Verification items for the finished model (mm, model axes). A direction names the side the tool comes from. Round coordinates to 2 decimals unless told otherwise and drop trailing zeros. Write each loop counter-clockwise with the first axis right and the second up, starting at its lowest first coordinate (ties: lowest second). Pieces come first, ordered by that corner, then holes. Notation, with made-up numbers: (63.25, 78) - (73.25, 78) arc R29 ccw to (73.25, 106) - close; hole circle Ø10 at (33, 79). An arc over 180 degrees is marked (long way). Answer as a JSON object with one key per item and string values. Group by question number.
1) Thickness scan on line 1 (Y direction, x = 34, z = 16.5); line 2 (X direction, y = -39, z = 21.5); line 3 (X direction, y = 39, z = 21.25). Record the ranges inside material, lowest first.
2) Go/stop test with flat-tipped pins: pin 1 Ø7 at (y, z) = (40, 12) entering from -X; pin 2 Ø1.9 at (y, z) = (-40.5, 14) entering from +X; pin 3 Ø12 at (x, y) = (20, -11) entering from +Z. Record where each tip stops, or that it passes through.
3) Set-up check for faces 1 (the flat face through (-1, 0, 15)), 2 (the flat face through (-40, 42, 15)), 3 (the flat face through (40, 42, 15)): record each of +Z, -Z, +X, -X, +Y, -Y from which the full face is reachable in a straight line by a thin tool's end or side.
4) Section check D-D (y = -14). Enter the section's corners in (x, z).
5) Mould release check, pull along Z, two halves, no side actions. Record for faces 4 (the cylindrical face through (59.47, -0.39, 7.4)), 5 (the cylindrical face through (29.514, -39.943, 20.304)), 6 (the flat face through (1, 1, 0)): +Z half, -Z half, draft (parallel to the pull), parting line (faces both ways), or undercut.
6) Section check C-C (x = 8). Enter the section's corners in (y, z).
7) Section check A-A (z = 18). Enter the section's corners in (x, y), then the cut area to 3 significant figures.
8) Section check B-B (x = -23). Enter the section's corners in (y, z).
```python
from build123d import *

# Parameters (mm, degrees)
SKETCH1_R               = 10.5
BOSS_EXTRUDE1_DEPTH     = 15
BOSS_EXTRUDE2_DEPTH     = 30
SKETCH2_R               = 2.25
CUT_EXTRUDE1_DEPTH      = 1
CUT_EXTRUDE1_DEPTH_BACK = 90.5


with BuildPart() as part:
    # Sketch1 → Boss-Extrude1 (new body)
    with BuildSketch(Plane.XY):
        with BuildLine():
            Line((-40.319533419, -35), (40.319533419, -35))
            ThreePointArc((40.319533419, -35), (42.786608734, -28.756118968), (47.370059804, -23.850562196))
            ThreePointArc((47.370059804, -23.850562196), (59.471288553, 0.00030559), (47.370059804, 23.851173376))
            ThreePointArc((47.370059804, 23.851173376), (42.786775017, 28.756467199), (40.31965015, 35))
            Line((40.31965015, 35), (-40.31965015, 35))
            ThreePointArc((-40.31965015, 35), (-42.786775017, 28.756467199), (-47.370059804, 23.851173376))
            ThreePointArc((-47.370059804, 23.851173376), (-59.471288553, 0.00030559), (-47.370059804, -23.850562196))
            ThreePointArc((-47.370059804, -23.850562196), (-42.786608734, -28.756118968), (-40.319533419, -35))
        make_face()
        with Locations((29.916288553, 0.00030559)):
            Circle(SKETCH1_R, mode=Mode.SUBTRACT)
        with Locations((-29.916288553, 0.00030559)):
            Circle(SKETCH1_R, mode=Mode.SUBTRACT)
    extrude(amount=BOSS_EXTRUDE1_DEPTH)

    # Sketch1_3 → Boss-Extrude2 (add)
    with BuildSketch(Plane.XY):
        with BuildLine():
            ThreePointArc((-40.31965015, 35), (-40.080090719, 36.681034549), (-40, 38.377162892))
            Line((-40, 38.377162892), (-40, 44.75))
            Line((-40, 44.75), (40, 44.75))
            Line((40, 44.75), (40, 38.377162892))
            ThreePointArc((40, 38.377162892), (40.080090719, 36.681034549), (40.31965015, 35))
            Line((40.31965015, 35), (-40.31965015, 35))
        make_face()
        with BuildLine():
            ThreePointArc((40.319533419, -35), (40.080061405, -36.6807331), (40, -38.376551713))
            Line((40, -38.376551713), (40, -44.75))
            Line((40, -44.75), (-40, -44.75))
            Line((-40, -44.75), (-40, -38.376551713))
            ThreePointArc((-40, -38.376551713), (-40.080061405, -36.6807331), (-40.319533419, -35))
            Line((-40.319533419, -35), (40.319533419, -35))
        make_face()
    extrude(amount=BOSS_EXTRUDE2_DEPTH)

    # Sketch2 → Cut-Extrude1 (cut, two sides)
    with BuildSketch(Plane.XZ.offset(44.75)) as cut_extrude1_sk:
        with Locations((-30.001288553, 22.5)):
            Circle(SKETCH2_R)
        with Locations((30.001288553, 22.5)):
            Circle(SKETCH2_R)
    extrude(amount=CUT_EXTRUDE1_DEPTH, mode=Mode.SUBTRACT)
    extrude(cut_extrude1_sk.sketch, amount=-CUT_EXTRUDE1_DEPTH_BACK, mode=Mode.SUBTRACT)


solid = part.part
```
Returned:
{
 "1": {"line 1": "-44.75 to -35, 35 to 44.75", "line 2": "-40 to -32.02, -27.99 to 27.99, 32.02 to 40", "line 3": "-40 to -31.87, -28.13 to 28.13, 31.87 to 40"},
 "2": {"pin 1": "x = -40.1", "pin 2": "x = 40", "pin 3": "z = 15"},
 "3": {"face 1": "+Z, +X, -X", "face 2": "+Z, -Z, -X, +Y", "face 3": "+Z, -Z, +X, +Y"},
 "4": {"outline": "(-55.94, 0) - (55.94, 0) - (55.94, 15) - (-55.94, 15) - close"},
 "5": {"face 4": "draft", "face 5": "undercut", "face 6": "-Z half"},
 "6": {"outline": "(-44.75, 0) - (44.75, 0) - (44.75, 30) - (35, 30) - (35, 15) - (-35, 15) - (-35, 30) - (-44.75, 30) - close"},
 "7": {"outline": "(-40.32, -35) arc R18 cw to (-40, -38.38) - (-40, -44.75) - (40, -44.75) - (40, -38.38) arc R18 cw to (40.32, -35) - close; (-40.32, 35) - (40.32, 35) arc R18 cw to (40, 38.38) - (40, 44.75) - (-40, 44.75) - (-40, 38.38) arc R18 cw to start", "area": "1,560 mm2"},
 "8": {"outline": "(-44.75, 0) - (-7.9, 0) - (-7.9, 15) - (-35, 15) - (-35, 30) - (-44.75, 30) - close; (7.9, 0) - (44.75, 0) - (44.75, 30) - (35, 30) - (35, 15) - (7.9, 15) - close"}
}
